Input: part model. Units: mm. Frame: model coordinates. Coordinates: 2 decimals unless noted, no trailing zeros. Write each loop counter-clockwise with the first axis right and the second up, starting at its lowest first coordinate (ties: lowest second). Pieces come first, ordered by that corner, then holes.
from build123d import *

# Parameters (mm, degrees)
SKETCH1_W          = 76.2
SKETCH1_H          = 6.35
BASE_EXTRUDE_DEPTH = 19.05
CUT_EXTRUDE1_DEPTH = 7.35
SKETCH3_R          = 2.38125
CUT_EXTRUDE2_DEPTH = 7.35


with BuildPart() as part:
    # Sketch1 → Base-Extrude (new body)
    with BuildSketch(Plane.XY):
        with Locations((38.1, 3.175)):
            Rectangle(SKETCH1_W, SKETCH1_H)
    extrude(amount=BASE_EXTRUDE_DEPTH)

    # Sketch2 → Cut-Extrude1 (cut, through all)
    with BuildSketch(Plane(origin=(0, 6.35, 0), x_dir=(-1, 0, 0), z_dir=(0, 1, 0))):
        with BuildLine():
            Line((-71.4375, 5.324869794), (-71.4375, 13.725130206))
            ThreePointArc((-71.4375, 13.725130206), (-60.325, 9.525), (-71.4375, 5.324869794))
        make_face()
    extrude(amount=-CUT_EXTRUDE1_DEPTH, mode=Mode.SUBTRACT)

    # Sketch3 → Cut-Extrude2 (cut, through all)
    with BuildSketch(Plane(origin=(0, 6.35, 0), x_dir=(-1, 0, 0), z_dir=(0, 1, 0))):
        with Locations((-9.525, 9.525)):
            Circle(SKETCH3_R)
    extrude(amount=-CUT_EXTRUDE2_DEPTH, mode=Mode.SUBTRACT)


solid = part.part
Item 1: Pin query (flat end, axial travel): pin 1 Ø4 at (x, z) = (9.525, 9.525) entering from -Y. Return the tip coordinate at first contact, or that it passes through.
Item 2: Section query B-B, the plane y = 3.5. State how many separate pieces and enclosed holes the cut face has, then the cut area to 3 significant figures.
Item 3: Section query C-C, the plane z = 10.25. Return loops of the section in (x, y), then the cut area to 3 significant figures.
Item 4: Material intervals for line 1 (X direction, y = 3, z = 9.25); line 2 (Z direction, x = 67, y = 5.25); line 3 (X direction, y = 4.75, z = 9), sorted ascending.
Item 5: Pull-direction query (Z, two-part tool) for faces 1 (the face through (38, 3, 19.05)), 2 (the face through (71.438, 3, 9)), 3 (the face through (8.24, 3.22, 11.53)), 4 (the face through (76.2, 3, 9)); classes: released by +Z, released by -Z, zero draft, split by the parting line, or undercut.
Item 6: Section query A-A, the plane x = 63.5. Return loops of the section in (y, z).
The answers:
1. pin 1: passes through
2. separate pieces: 1
2. enclosed holes: 2
2. area: 1,320 mm2
3. outline: (0, 0) - (7.26, 0) - (7.26, 6.35) - (0, 6.35) - close; (11.79, 0) - (60.37, 0) - (60.37, 6.35) - (11.79, 6.35) - close; (71.44, 0) - (76.2, 0) - (76.2, 6.35) - (71.44, 6.35) - close
3. area: 385 mm2
4. line 1: x = 0 to 7.16, 11.89 to 60.33, 71.44 to 76.2
4. line 2: z = 0 to 3.18, 15.87 to 19.05
4. line 3: x = 0 to 7.2, 11.85 to 60.35, 71.44 to 76.2
5. face 1: released by +Z
5. face 2: undercut
5. face 3: undercut
5. face 4: zero draft
6. outline: (0, 0) - (6.35, 0) - (6.35, 4.03) - (0, 4.03) - close; (0, 15.02) - (6.35, 15.02) - (6.35, 19.05) - (0, 19.05) - close
